```python
from build123d import *

# Parameters (mm, degrees)
SKETCH1_R                     = 2.15265
SKETCH1_R_2                   = 9.525
SKETCH1_R_3                   = 2.4892
BOSS_EXTRUDE1_DEPTH           = 1.5875
CUT_EXTRUDE1_DEPTH            = 2.54
F_13_64_0_18_DIAMETER_HOLE1_D = 4.572
SKETCH7_W                     = 317.5
SKETCH7_H                     = 35.56
CUT_EXTRUDE2_DEPTH            = 288.517243505


with BuildPart() as part:
    # Sketch1 → Boss-Extrude1 (new body)
    # profile 1 of 21: a face of its own
    with BuildSketch(Plane(origin=(0, 0, 0), x_dir=(1, 0, 0), z_dir=(0, 1, 0))):
        with BuildLine():
            Line((-97.234377561, 239.7125), (-158.75, 239.7125))
            Line((-158.75, 239.7125), (-158.75, -239.7125))
            Line((-158.75, -239.7125), (158.75, -239.7125))
            Line((158.75, -239.7125), (158.75, 239.7125))
            Line((158.75, 239.7125), (97.234377561, 239.7125))
            ThreePointArc((97.234377561, 239.7125), (97.124777, 233.170194434), (91.44, 229.930273932))
            Line((91.44, 229.930273932), (-91.44, 229.930273932))
            ThreePointArc((-91.44, 229.930273932), (-97.124777, 233.170194434), (-97.234377561, 239.7125))
        make_face()
        with Locations(Location((-147.828, -193.4845, 0), (0, 0, 270))):
            Circle(SKETCH1_R, mode=Mode.SUBTRACT)
        with Locations((-104.14, -4.1275)):
            Circle(SKETCH1_R_2, mode=Mode.SUBTRACT)
        with BuildLine():
            ThreePointArc((-97.79, -204.7875), (-104.14, -198.4375), (-97.79, -192.0875))
            Line((-97.79, -192.0875), (97.79, -192.0875))
            ThreePointArc((97.79, -192.0875), (104.14, -198.4375), (97.79, -204.7875))
            Line((97.79, -204.7875), (-97.79, -204.7875))
        make_face(mode=Mode.SUBTRACT)
        with Locations(Location((147.828, -193.4845, 0), (0, 0, 270))):
            Circle(SKETCH1_R, mode=Mode.SUBTRACT)
        with Locations((104.14, -4.1275)):
            Circle(SKETCH1_R_2, mode=Mode.SUBTRACT)
        with Locations((-126.365, 30.1625)):
            Circle(SKETCH1_R, mode=Mode.SUBTRACT)
        with Locations((-126.365, 49.2125)):
            Circle(SKETCH1_R, mode=Mode.SUBTRACT)
        with Locations((-104.14, 40.0685)):
            Circle(SKETCH1_R_2, mode=Mode.SUBTRACT)
        with Locations((-104.14, 84.2645)):
            Circle(SKETCH1_R_3, mode=Mode.SUBTRACT)
        with Locations((-126.365, 163.5125)):
            Circle(SKETCH1_R, mode=Mode.SUBTRACT)
        with Locations((-126.365, 182.5625)):
            Circle(SKETCH1_R, mode=Mode.SUBTRACT)
        with Locations((-104.14, 128.4605)):
            Circle(SKETCH1_R_2, mode=Mode.SUBTRACT)
        with Locations((-104.14, 172.6565)):
            Circle(SKETCH1_R_2, mode=Mode.SUBTRACT)
        with Locations(Location((-147.828, 228.7905, 0), (0, 0, 270))):
            Circle(SKETCH1_R, mode=Mode.SUBTRACT)
        with Locations((-104.14, 216.8525)):
            Circle(SKETCH1_R_2, mode=Mode.SUBTRACT)
        with Locations((104.14, 40.0685)):
            Circle(SKETCH1_R_2, mode=Mode.SUBTRACT)
        with Locations((126.365, 30.1625)):
            Circle(SKETCH1_R, mode=Mode.SUBTRACT)
        with Locations((126.365, 49.2125)):
            Circle(SKETCH1_R, mode=Mode.SUBTRACT)
        with Locations((104.14, 84.2645)):
            Circle(SKETCH1_R_3, mode=Mode.SUBTRACT)
        with Locations((104.14, 128.4605)):
            Circle(SKETCH1_R_2, mode=Mode.SUBTRACT)
        with Locations((104.14, 172.6565)):
            Circle(SKETCH1_R_2, mode=Mode.SUBTRACT)
        with Locations((126.365, 163.5125)):
            Circle(SKETCH1_R, mode=Mode.SUBTRACT)
        with Locations((126.365, 182.5625)):
            Circle(SKETCH1_R, mode=Mode.SUBTRACT)
        with Locations((104.14, 216.8525)):
            Circle(SKETCH1_R_2, mode=Mode.SUBTRACT)
        with Locations(Location((147.828, 228.7905, 0), (0, 0, 270))):
            Circle(SKETCH1_R, mode=Mode.SUBTRACT)
    # profile 2 of 21: a face of its own
    with BuildSketch(Plane(origin=(0, 0, 0), x_dir=(1, 0, 0), z_dir=(0, 1, 0))):
        with Locations((-104.14, 216.8525)):
            Circle(SKETCH1_R_2)
    # profile 3 of 21: a face of its own
    with BuildSketch(Plane(origin=(0, 0, 0), x_dir=(1, 0, 0), z_dir=(0, 1, 0))):
        with Locations((-104.14, 172.6565)):
            Circle(SKETCH1_R_2)
    # profile 4 of 21: a face of its own
    with BuildSketch(Plane(origin=(0, 0, 0), x_dir=(1, 0, 0), z_dir=(0, 1, 0))):
        with Locations((-104.14, 128.4605)):
            Circle(SKETCH1_R_2)
    # profile 5 of 21: a face of its own
    with BuildSketch(Plane(origin=(0, 0, 0), x_dir=(1, 0, 0), z_dir=(0, 1, 0))):
        with Locations((-104.14, -4.1275)):
            Circle(SKETCH1_R_2)
    # profile 6 of 21: a face of its own
    with BuildSketch(Plane(origin=(0, 0, 0), x_dir=(1, 0, 0), z_dir=(0, 1, 0))):
        with Locations((-104.14, 40.0685)):
            Circle(SKETCH1_R_2)
    # profile 7 of 21: a face of its own
    with BuildSketch(Plane(origin=(0, 0, 0), x_dir=(1, 0, 0), z_dir=(0, 1, 0))):
        with Locations((104.14, 40.0685)):
            Circle(SKETCH1_R_2)
    # profile 8 of 21: a face of its own
    with BuildSketch(Plane(origin=(0, 0, 0), x_dir=(1, 0, 0), z_dir=(0, 1, 0))):
        with Locations((104.14, -4.1275)):
            Circle(SKETCH1_R_2)
    # profile 9 of 21: a face of its own
    with BuildSketch(Plane(origin=(0, 0, 0), x_dir=(1, 0, 0), z_dir=(0, 1, 0))):
        with Locations((104.14, 172.6565)):
            Circle(SKETCH1_R_2)
    # profile 10 of 21: a face of its own
    with BuildSketch(Plane(origin=(0, 0, 0), x_dir=(1, 0, 0), z_dir=(0, 1, 0))):
        with Locations((104.14, 216.8525)):
            Circle(SKETCH1_R_2)
    # profile 11 of 21: a face of its own
    with BuildSketch(Plane(origin=(0, 0, 0), x_dir=(1, 0, 0), z_dir=(0, 1, 0))):
        with Locations((104.14, 128.4605)):
            Circle(SKETCH1_R_2)
    # profile 12 of 21: a face of its own
    with BuildSketch(Plane(origin=(0, 0, 0), x_dir=(1, 0, 0), z_dir=(0, 1, 0))):
        with Locations((126.365, 30.1625)):
            Circle(SKETCH1_R)
    # profile 13 of 21: a face of its own
    with BuildSketch(Plane(origin=(0, 0, 0), x_dir=(1, 0, 0), z_dir=(0, 1, 0))):
        with Locations((126.365, 49.2125)):
            Circle(SKETCH1_R)
    # profile 14 of 21: a face of its own
    with BuildSketch(Plane(origin=(0, 0, 0), x_dir=(1, 0, 0), z_dir=(0, 1, 0))):
        with Locations((126.365, 163.5125)):
            Circle(SKETCH1_R)
    # profile 15 of 21: a face of its own
    with BuildSketch(Plane(origin=(0, 0, 0), x_dir=(1, 0, 0), z_dir=(0, 1, 0))):
        with Locations((126.365, 182.5625)):
            Circle(SKETCH1_R)
    # profile 16 of 21: a face of its own
    with BuildSketch(Plane(origin=(0, 0, 0), x_dir=(1, 0, 0), z_dir=(0, 1, 0))):
        with Locations((-126.365, 163.5125)):
            Circle(SKETCH1_R)
    # profile 17 of 21: a face of its own
    with BuildSketch(Plane(origin=(0, 0, 0), x_dir=(1, 0, 0), z_dir=(0, 1, 0))):
        with Locations((-126.365, 182.5625)):
            Circle(SKETCH1_R)
    # profile 18 of 21: a face of its own
    with BuildSketch(Plane(origin=(0, 0, 0), x_dir=(1, 0, 0), z_dir=(0, 1, 0))):
        with Locations((-126.365, 49.2125)):
            Circle(SKETCH1_R)
    # profile 19 of 21: a face of its own
    with BuildSketch(Plane(origin=(0, 0, 0), x_dir=(1, 0, 0), z_dir=(0, 1, 0))):
        with Locations((-126.365, 30.1625)):
            Circle(SKETCH1_R)
    # profile 20 of 21: a face of its own
    with BuildSketch(Plane(origin=(0, 0, 0), x_dir=(1, 0, 0), z_dir=(0, 1, 0))):
        with Locations((104.14, 84.2645)):
            Circle(SKETCH1_R_3)
    # profile 21 of 21: a face of its own
    with BuildSketch(Plane(origin=(0, 0, 0), x_dir=(1, 0, 0), z_dir=(0, 1, 0))):
        with Locations((-104.14, 84.2645)):
            Circle(SKETCH1_R_3)
    extrude(amount=BOSS_EXTRUDE1_DEPTH)

    # Sketch2 → Cut-Extrude1 (cut)
    with BuildSketch(Plane(origin=(0, 1.5875, 0), x_dir=(1, 0, 0), z_dir=(0, 1, 0))):
        Polygon((-39.37, 230.1875), (-44.45, 230.1875), (-44.45, 116.18638997), (-44.45, 111.10638997), (-39.37, 111.10638997), (-24.13, 111.10638997), (-24.13, 80.773994761), (-24.13, 75.693994761), (-44.45, 75.693994761), (-44.45, 69.693451711), (-19.05, 69.693451711), (-19.05, 75.693994761), (-19.05, 111.10638997), (-19.05, 116.18638997), (-39.37, 116.18638997), align=None)
        Polygon((36.83, 230.1875), (31.75, 230.1875), (31.75, 116.18638997), (12.478280381, 116.18638997), (12.478280381, 111.10638997), (12.478280381, 97.725538056), (12.478280381, 95.043026282), (27.466923788, 95.043026282), (32.944773159, 95.043026282), (32.944773159, 94.327747899), (32.944773159, 54.465469302), (19.338923788, 54.465469302), (14.258923788, 54.465469302), (14.258923788, 49.385469302), (14.258923788, 39.311344325), (6.047836395, 39.311344325), (0.967836395, 39.311344325), (0.967836395, 34.231344325), (0.967836395, 9.126281939), (0.967836395, 4.046281939), (6.047836395, 4.046281939), (13.97, 4.046281939), (19.05, 4.046281939), (19.05, 9.126281939), (19.05, 16.514356244), (32.944773159, 16.514356244), (32.944773159, -1.068708856), (26.67, -1.068708856), (26.67, -6.148708856), (26.67, -26.035), (31.75, -26.035), (31.75, -6.148708856), (32.944773159, -6.148708856), (38.024773159, -6.148708856), (38.024773159, -1.068708856), (38.024773159, 16.514356244), (38.024773159, 21.594356244), (19.05, 21.594356244), (13.97, 21.594356244), (13.97, 16.514356244), (13.97, 9.126281939), (6.047836395, 9.126281939), (6.047836395, 34.231344325), (14.258923788, 34.231344325), (19.338923788, 34.231344325), (19.338923788, 39.311344325), (19.338923788, 49.385469302), (38.024773159, 49.385469302), (38.024773159, 54.465469302), (38.024773159, 94.327747899), (38.024773159, 95.043026282), (38.024773159, 100.123026282), (19.090989095, 100.123026282), (17.558280381, 100.123026282), (17.558280381, 111.10638997), (36.83, 111.10638997), (36.83, 116.18638997), align=None)
    extrude(amount=-CUT_EXTRUDE1_DEPTH, mode=Mode.SUBTRACT)

    # 13/64 (0.18) Diameter Hole1 (through all)
    with Locations(Plane(origin=(0, 0, 0), x_dir=(-1, 0, 0), z_dir=(0, -1, 0))):
        with Locations((-82.55, 194.6275), (12.7, 194.6275), (-82.55, 171.7675), (12.7, 171.7675)):
            Hole(F_13_64_0_18_DIAMETER_HOLE1_D / 2)

    # Sketch7 → Cut-Extrude2 (cut, through all)
    with BuildSketch(Plane(origin=(0, 1.5875, 0), x_dir=(1, 0, 0), z_dir=(0, 1, 0))):
        with Locations((0, -221.9325)):
            Rectangle(SKETCH7_W, SKETCH7_H)
    extrude(amount=-CUT_EXTRUDE2_DEPTH, mode=Mode.SUBTRACT)


solid = part.part
```
Check sheet for the modelled part. Datum: model origin and axes. Units: mm. Round coordinates to 2 decimals unless told otherwise and drop trailing zeros. Loops run counter-clockwise (first coordinate to the right, second up) from the corner with the lowest first, then second, coordinate; pieces in that order, holes last. Notation, with made-up numbers: (-24, 1) - (7, 1) arc R14 ccw to (7, 11) - close; hole circle Ø7 at (57.25, 87). An arc over 180 degrees is marked (long way). Answer as a JSON object with one key per item and string values. Group by question number.
Q1. Gauge pin test, flat ends, axial feed: P1, Ø0.8, axis at x = -61, y = 0.5, coming from the -Z side; P2, Ø3.5, axis at x = -147.83, z = 193.48, coming from the -Y side. Record the tip position at first contact, or that the pin passes through.
Q2. Scan lines: line 1 along X through (y, z) = (0.15, -88.5); line 2 along X through (y, z) = (1.35, -178.5); line 3 along Z through (x, y) = (82.55, 0.6). Record each from-to range of solid material in increasing order. Write a range as [from, to].
Q3. Sectioned sample at B-B, the plane y = 1.3. Count the separate pieces of the cut face and the enclosed holes in it, plus the area to 3 significant figures.
Q4. Sectioned sample at A-A, the plane z = -146. Enter the section's corners in (x, y), plus the area to 3 significant figures.
Solution:
{
 "1": {"P1": "stops at z = -229.93", "P2": "passes through"},
 "2": {"line 1": "x = [-158.75, -24.13], [-19.05, 32.94], [38.02, 158.75]", "line 2": "x = [-158.75, -44.45], [-39.37, 31.75], [36.83, 158.75]", "line 3": "z = [-229.93, -196.91], [-192.34, -174.05], [-169.48, 192.09]"},
 "3": {"separate pieces": "1", "enclosed holes": "8", "area": "133,000 mm²"},
 "4": {"outline": "(-158.75, 0) - (-44.45, 0) - (-44.45, 1.59) - (-158.75, 1.59) - close; (-39.37, 0) - (31.75, 0) - (31.75, 1.59) - (-39.37, 1.59) - close; (36.83, 0) - (158.75, 0) - (158.75, 1.59) - (36.83, 1.59) - close", "area": "488 mm²"}
}
